Study the drawing (mm; zero at the part's minimum x, y, z) and answer. A direction names the side the tool comes from. Give positions to 0.01 mm unless a question says otherwise; leave off trailing zeros. Write each loop counter-clockwise with the first axis right and the second up, starting at its lowest first coordinate (ties: lowest second). Pieces come first, ordered by that corner, then holes. Notation, with made-up numbers: (64, 7) - (111, 7) arc R20 cw to (111, 30) - close; hole circle Ø2 at (65.5, 33.25). An arc over 180 degrees is marked (long way). Write each question's results on one line, items separated by ' | '. Start each with the question number.
Q1. For the marked faces 1, 2 and 3, determine the directions among +Z, -Z, +X, -X, +Y, -Y from which every point of the face is accessible in a straight line to the end or side of a thin tool.
Q2. Section C-C (y = 19.92) is taken. Determine the outline of the cut face in (x, z) (3 decimals).
Q3. Flat-ended cylindrical pins translate along their axes: pin 1 Ø2.5 at (y, z) = (18.5, 2) entering from -X; pin 2 Ø16.5 at (y, z) = (7.5, 17.5) entering from -X; pin 3 Ø12 at (x, y) = (49, 9.5) entering from +Z (3 decimals). Find the tip coordinate at first contact, or state that the pin passes through.
Q4. Section A-A (y = 54.92) is taken. Determine the outline of the cut face in (x, z) (3 decimals).
Q5. Section D-D (z = 30) is taken. Determine the outline of the cut face in (x, y), plus the area to 3 significant figures.
Q6. Find the intervals of material crossed by probe 1 along X at (y, z) = (5.5, 12) (3 decimals); probe 2 along Z at (x, y) = (37.5, 12.5) (3 decimals); probe 3 along Z at (x, y) = (14.5, 21) (3 decimals), in increasing order.
Q7. Section B-B (x = 7.5) is taken. Determine the outline of the cut face in (y, z) (3 decimals), plus the area to 3 significant figures.
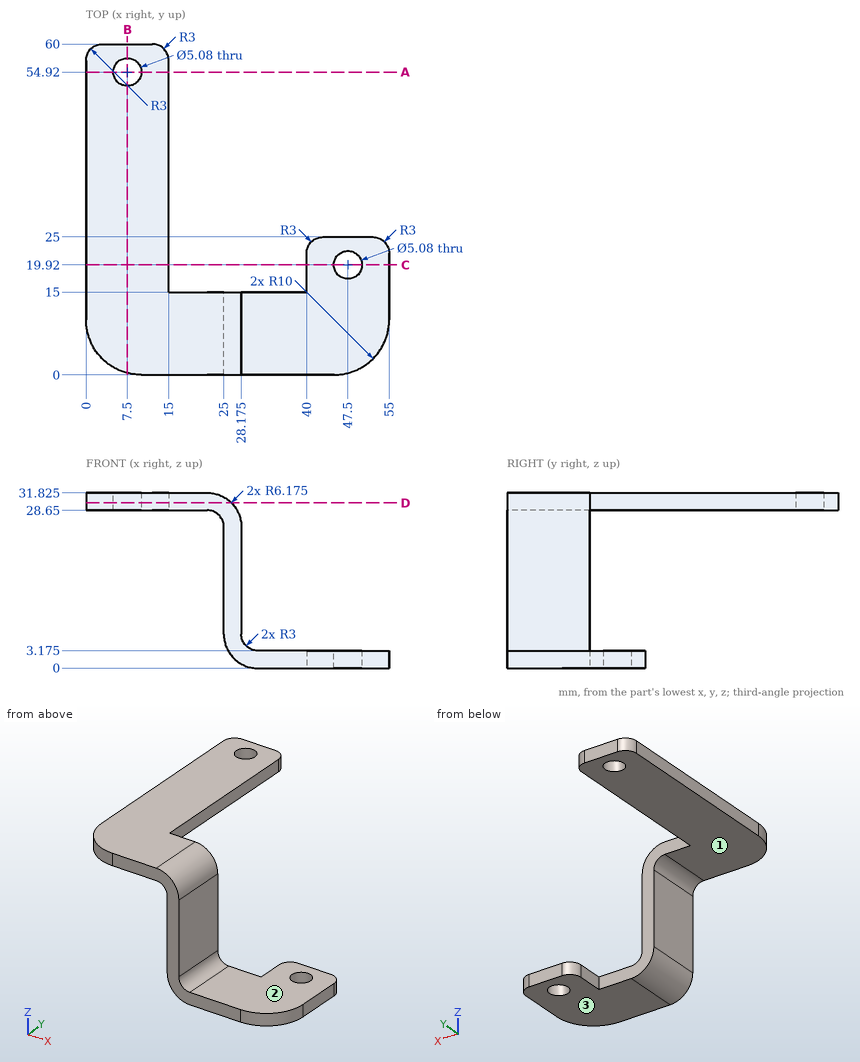
Answers below:
1) face 1: -Z, -X, +Y, -Y | face 2: +Z, +X, +Y, -Y | face 3: -Z, +X, -X, +Y, -Y
2) outline: (0, 28.65) - (15, 28.65) - (15, 31.825) - (0, 31.825) - close; (40, 0) - (44.96, 0) - (44.96, 3.175) - (40, 3.175) - close; (50.04, 0) - (55, 0) - (55, 3.175) - (50.04, 3.175) - close
3) pin 1: stops at x = 40 | pin 2: stops at x = 25 | pin 3: stops at z = 3.175
4) outline: (0, 28.65) - (4.96, 28.65) - (4.96, 31.825) - (0, 31.825) - close; (10.04, 28.65) - (15, 28.65) - (15, 31.825) - (10.04, 31.825) - close
5) outline: (0, 10) arc R10 ccw to (10, 0) - (26.38, 0) - (26.38, 15) - (15, 15) - (15, 57) arc R3 ccw to (12, 60) - (3, 60) arc R3 ccw to (0, 57) - close; hole circle Ø5.08 at (7.5, 54.92) | area: 1,030 mm2
6) probe 1: x = 25 to 28.175 | probe 2: z = 0 to 3.175 | probe 3: z = 28.65 to 31.825
7) outline: (0.318, 28.65) - (52.38, 28.65) - (52.38, 31.825) - (0.318, 31.825) - close; (57.46, 28.65) - (60, 28.65) - (60, 31.825) - (57.46, 31.825) - close | area: 173 mm2
